from build123d import *

# Parameters (mm, degrees)
SKETCH_1_R      = 90
SKETCH_1_R_2    = 80
EXTRUDE_1_DEPTH = 2
SKETCH_1_3_R    = 92.5
SKETCH_1_3_R_2  = 90
SKETCH_1_3_R_3  = 80
SKETCH_1_3_R_4  = 77.5
EXTRUDE_2_DEPTH = 12


with BuildPart() as part:
    # Sketch 1 → Extrude 1 (new body)
    with BuildSketch(Plane(origin=(0, 0, 0), x_dir=(1, 0, 0), z_dir=(0, 1, 0))):
        with Locations(Location((0, 0, 0), (0, 0, 270))):
            Circle(SKETCH_1_R)
        with Locations(Location((0, 0, 0), (0, 0, 270))):
            Circle(SKETCH_1_R_2, mode=Mode.SUBTRACT)
    extrude(amount=EXTRUDE_1_DEPTH)

    # Sketch 1_3 → Extrude 2 (add)
    # profile 1 of 2: a face of its own
    with BuildSketch(Plane(origin=(0, 0, 0), x_dir=(1, 0, 0), z_dir=(0, 1, 0))):
        with Locations(Location((0, 0, 0), (0, 0, 270))):
            Circle(SKETCH_1_3_R)
        with Locations(Location((0, 0, 0), (0, 0, 270))):
            Circle(SKETCH_1_3_R_2, mode=Mode.SUBTRACT)
    # profile 2 of 2: a face of its own
    with BuildSketch(Plane(origin=(0, 0, 0), x_dir=(1, 0, 0), z_dir=(0, 1, 0))):
        with Locations(Location((0, 0, 0), (0, 0, 270))):
            Circle(SKETCH_1_3_R_3)
        with Locations(Location((0, 0, 0), (0, 0, 270))):
            Circle(SKETCH_1_3_R_4, mode=Mode.SUBTRACT)
    extrude(amount=EXTRUDE_2_DEPTH)


solid = part.part
Work out the finished part from the listing and answer in its coordinate system (mm). A direction names the side the tool comes from. Round coordinates to 2 decimals unless told otherwise and drop trailing zeros. Write each loop counter-clockwise with the first axis right and the second up, starting at its lowest first coordinate (ties: lowest second). Pieces come first, ordered by that corner, then holes. Notation, with made-up numbers: (87.25, -13.75) - (114.25, -13.75) arc R16 cw to (114.25, 9.25) - close; hole circle Ø2 at (16.5, -6). An arc over 180 degrees is marked (long way). Answer in a Markdown table with one row per item. Add a question column.
1. Given pin 1 (12 mm diameter, centred on x = 69, z = 32.5, fed in from +Y); pin 2 (6 mm diameter, centred on x = -48.5, y = 3.5, fed in from +Z); pin 3 (6 mm diameter, centred on x = -73, z = -46, fed in from +Y); pin 4 (1.5 mm diameter, centred on x = 16, y = 2.5, fed in from -Z), each flat-ended and moving along its own axis, determine where each tip first touches the part or whether it passes through.
2. A cutting plane is placed at B-B, the plane z = 0. Determine the outline of the cut face in (x, y).
3. The mould has two halves that part along Z. Classify faces 3 (the flat face through (66, 12, -42)), 4 (the cylindrical face through (-34.471, 6.93, 83.137)), 5 (the cylindrical face through (-90.3, 5.92, -20.05)): +Z half, -Z half, draft (parallel to the pull), parting line (faces both ways), or undercut.
4. Find the intervals of material crossed by line 1 along X through (y, z) = (9, 0); line 2 along Z through (x, y) = (16.5, 5); line 3 along Z through (x, y) = (41, 8.5), in increasing order. Write a range as from..to.
5. A cutting plane is placed at C-C, the plane y = 9.5. Determine the outline of the cut face in (x, z), and give its area (3 significant figures).
6. For faces 1 (the cylindrical face through (-78.1, 6.93, -17.34)), 2 (the flat face through (-75, 0, -21)), determine the directions among +Z, -Z, +X, -X, +Y, -Y from which every point of the face is accessible in a straight line to the end or side of a thin tool.
7. A cutting plane is placed at A-A, the plane x = 0. Determine the outline of the cut face in (y, z).
Worked out:
| question | item | result |
|---|---|---|
| 1 | pin 1 | y = 12 |
| 1 | pin 2 | z = 80.54 |
| 1 | pin 3 | y = 2 |
| 1 | pin 4 | z = -91.23 |
| 2 | outline | (-92.5, 0) - (-77.5, 0) - (-77.5, 12) - (-80, 12) - (-80, 2) - (-90, 2) - (-90, 12) - (-92.5, 12) - close; (77.5, 0) - (92.5, 0) - (92.5, 12) - (90, 12) - (90, 2) - (80, 2) - (80, 12) - (77.5, 12) - close |
| 3 | face 3 | draft |
| 3 | face 4 | undercut |
| 3 | face 5 | parting line |
| 4 | line 1 | -92.5..-90, -80..-77.5, 77.5..80, 90..92.5 |
| 4 | line 2 | -91.02..-88.47, -78.28..-75.72, 75.72..78.28, 88.47..91.02 |
| 4 | line 3 | -82.92..-80.12, -68.69..-65.77, 65.77..68.69, 80.12..82.92 |
| 5 | outline | circle Ø185 at (0, 0); circle Ø160 at (0, 0); hole circle Ø180 at (0, 0); hole circle Ø155 at (0, 0) |
| 5 | area | 2,670 mm^2 |
| 6 | face 1 | +Y |
| 6 | face 2 | +Z, -Z, +X, -X, -Y |
| 7 | outline | (0, -92.5) - (12, -92.5) - (12, -90) - (2, -90) - (2, -80) - (12, -80) - (12, -77.5) - (0, -77.5) - close; (0, 77.5) - (12, 77.5) - (12, 80) - (2, 80) - (2, 90) - (12, 90) - (12, 92.5) - (0, 92.5) - close |
